Verification items for the finished model (mm, model axes). A direction names the side the tool comes from. Coordinates: 2 decimals unless noted, no trailing zeros. Write each loop counter-clockwise with the first axis right and the second up, starting at its lowest first coordinate (ties: lowest second). Pieces come first, ordered by that corner, then holes. Notation, with made-up numbers: M 70.5,37.25 L 95.5,37.25 A23 cw 95.5,54.25 Z; hole C 25.25,60 d1. An arc over 180 degrees is marked long. Answer in a Markdown table with one row per item.
from build123d import *

# Parameters (mm, degrees)
SKETCH1_R           = 1.5
BOSS_EXTRUDE1_DEPTH = 3


with BuildPart() as part:
    # Sketch1 → Boss-Extrude1 (new body)
    with BuildSketch(Plane(origin=(0, 0, 0), x_dir=(1, 0, 0), z_dir=(0, 1, 0))):
        with BuildLine():
            Line((0, 0), (0, 10.5))
            ThreePointArc((0, 10.5), (0.732233047, 12.267766953), (2.5, 13))
            Line((2.5, 13), (12.5, 13))
            ThreePointArc((12.5, 13), (14.267766953, 12.267766953), (15, 10.5))
            Line((15, 10.5), (15, 0))
            Line((15, 0), (10, 0))
            Line((10, 0), (10, 3))
            Line((10, 3), (5, 3))
            Line((5, 3), (5, 0))
            Line((5, 0), (0, 0))
        make_face()
        with Locations(Location((7.5, 8, 0), (0, 0, 270))):
            Circle(SKETCH1_R, mode=Mode.SUBTRACT)
    extrude(amount=BOSS_EXTRUDE1_DEPTH)


solid = part.part
1) Sectioned sample at A-A (y = 0.7). Record the cut outline in (x, z), then the cut area to 3 significant figures.
Response values:
| item | result |
|---|---|
| outline | M 0,-10.5 A2.5 ccw 2.5,-13 L 12.5,-13 A2.5 ccw 15,-10.5 L 15,0 L 10,0 L 10,-3 L 5,-3 L 5,0 L 0,0 Z; hole C 7.5,-8 d3 |
| area | 170 mm² |
2) Release check for a two-part mould opening along X. For faces 3 (the face through (6, 0, -7)), 4 (the face through (0.713, 1.479, -12.248)), 5 (the face through (15, 1, -5)), 6 (the face through (10, 1, -1)) record: +X half, -X half, draft (parallel to the pull), parting line (faces both ways), or undercut.
Response values:
| item | result |
|---|---|
| face 3 | draft |
| face 4 | -X half |
| face 5 | +X half |
| face 6 | undercut |
3) Depth check by flat-ended pin: pin 1 (1.5 mm diameter, centred on x = 7, y = 2, fed in from +Z); pin 2 (1 mm diameter, centred on x = 4.5, z = -8, fed in from -Y); pin 3 (2.5 mm diameter, centred on x = 7.5, z = -8, fed in from +Y). Enter the tip coordinate at first touch or a pass-through.
Response values:
| item | result |
|---|---|
| pin 1 | stops at z = -3 |
| pin 2 | stops at y = 0 |
| pin 3 | passes through |
4) Sectioned sample at C-C (x = 7.5). Record the cut outline in (y, z).
Response values:
| item | result |
|---|---|
| outline | M 0,-13 L 3,-13 L 3,-9.5 L 0,-9.5 Z; M 0,-6.5 L 3,-6.5 L 3,-3 L 0,-3 Z |
5) Thickness scan on L1, parallel to X at y = 1.2, z = -8; L2, parallel to Z at x = 9.75, y = 2.2; L3, parallel to Z at x = 13, y = 1.45. Record the ranges inside material, lowest first. Write a range as [from, to].
Response values:
| item | result |
|---|---|
| L1 | x = [0, 6], [9, 15] |
| L2 | z = [-13, -3] |
| L3 | z = [-12.95, 0] |
6) Tool access check on faces 1 (the face through (7, 1, -13)), 2 (the face through (8, 1, -3)). Record the directions out of +Z, -Z, +X, -X, +Y, -Y that give a thin tool (end or side, any length) a straight path to the whole face; none if there is none.
Response values:
| item | result |
|---|---|
| face 1 | -Z, +X, -X, +Y, -Y |
| face 2 | +Z, +Y, -Y |
7) Sectioned sample at B-B (z = -1.5). Record the cut outline in (x, y).
Response values:
| item | result |
|---|---|
| outline | M 0,0 L 5,0 L 5,3 L 0,3 Z; M 10,0 L 15,0 L 15,3 L 10,3 Z |
